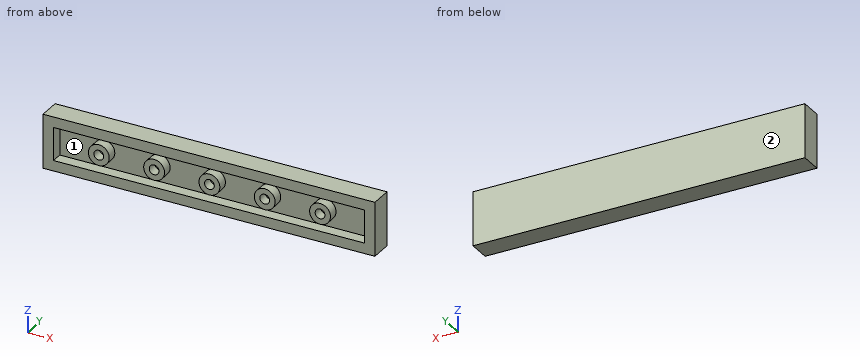
```python
from build123d import *

# Parameters (mm, degrees)
SKETCH1_W           = 47.75
SKETCH1_H           = 7.75
BOSS_EXTRUDE1_DEPTH = 3.15
SHELL1_T            = -1.5
SKETCH2_R           = 1.5
SKETCH2_R_2         = 0.7
BOSS_EXTRUDE2_DEPTH = 1.45


with BuildPart() as part:
    # Sketch1 → Boss-Extrude1 (new body)
    with BuildSketch(Plane(origin=(0, 0, 0), x_dir=(1, 0, 0), z_dir=(0, 1, 0))):
        Rectangle(SKETCH1_W, SKETCH1_H)
    extrude(amount=-BOSS_EXTRUDE1_DEPTH)

    # Shell1
    shell1_openings = [part.faces().sort_by_distance(p)[0] for p in [
        (0, -3.15, 0),
    ]]
    offset(amount=SHELL1_T, openings=shell1_openings, kind=Kind.INTERSECTION)

    # Sketch2 → Boss-Extrude2 (add)
    # profile 1 of 5: a face of its own
    with BuildSketch(Plane.XZ.offset(1.5)):
        with Locations(Location((-15.958333333, 0, 0), (0, 0, 90))):
            Circle(SKETCH2_R)
        with Locations(Location((-15.958333333, 0, 0), (0, 0, 90))):
            Circle(SKETCH2_R_2, mode=Mode.SUBTRACT)
    # profile 2 of 5: a face of its own
    with BuildSketch(Plane.XZ.offset(1.5)):
        with Locations(Location((-8, 0, 0), (0, 0, 90))):
            Circle(SKETCH2_R)
        with Locations(Location((-8, 0, 0), (0, 0, 90))):
            Circle(SKETCH2_R_2, mode=Mode.SUBTRACT)
    # profile 3 of 5: a face of its own
    with BuildSketch(Plane.XZ.offset(1.5)):
        with Locations(Location((-0.041666667, 0, 0), (0, 0, 90))):
            Circle(SKETCH2_R)
        with Locations(Location((-0.041666667, 0, 0), (0, 0, 90))):
            Circle(SKETCH2_R_2, mode=Mode.SUBTRACT)
    # profile 4 of 5: a face of its own
    with BuildSketch(Plane.XZ.offset(1.5)):
        with Locations(Location((7.916666667, 0, 0), (0, 0, 90))):
            Circle(SKETCH2_R)
        with Locations(Location((7.916666667, 0, 0), (0, 0, 90))):
            Circle(SKETCH2_R_2, mode=Mode.SUBTRACT)
    # profile 5 of 5: a face of its own
    with BuildSketch(Plane.XZ.offset(1.5)):
        with Locations(Location((15.875, 0, 0), (0, 0, 90))):
            Circle(SKETCH2_R)
        with Locations(Location((15.875, 0, 0), (0, 0, 90))):
            Circle(SKETCH2_R_2, mode=Mode.SUBTRACT)
    extrude(amount=BOSS_EXTRUDE2_DEPTH)


solid = part.part
```
For this review, take the finished solid that the model builds, in its own axes (mm). Face numbers are marked on the shaded views. Coordinates: 2 decimals unless noted, no trailing zeros. Loops run counter-clockwise (first coordinate to the right, second up) from the corner with the lowest first, then second, coordinate; pieces in that order, holes last. Notation, with made-up numbers: (48.25, 68.5) -> (105.25, 68.5) arc R21 cw to (105.25, 90.5) -> close; hole circle Ø3 at (68, 25.5). An arc over 180 degrees is marked (long way). Return JSON: item names as keys, results as strings. Group by question number.
(1) Mouldability with a two-part tool opening along X and no side actions: class the marked faces 1 and 2 as pulls with the +X half, pulls with the -X half, needs draft (parallel to the pull), parting line crosses it, or undercut.
(2) To check wall thickness, follow L1, parallel to Z at x = 0, y = -1.95 (3 decimals); L2, parallel to Z at x = -16.5, y = -2.3 (3 decimals); L3, parallel to X at y = -2.8, z = -2.25 (3 decimals). State the ranges of each line that lie inside material, in increasing order.
(3) Consider section B-B, the plane x = -8. Give the boundary of the cut face in (y, z) (3 decimals).
(4) Consider section A-A, the plane x = -13. Give the boundary of the cut face in (y, z) (3 decimals).
(5) For pin 1 Ø1.1 at (x, z) = (15.875, 0) entering from -Y; pin 2 Ø0.9 at (x, z) = (7.5, 0) entering from -Y, all flat-tipped, find the tip position at first contact; note any pin that passes through.
Results below:
{
 "1": {"face 1": "undercut", "face 2": "needs draft"},
 "2": {"L1": "z = -3.875 to -2.375, -1.499 to -0.699, 0.699 to 1.499, 2.375 to 3.875", "L2": "z = -3.875 to -2.375, -1.399 to -0.443, 0.443 to 1.399, 2.375 to 3.875", "L3": "x = -23.875 to -22.375, 22.375 to 23.875"},
 "3": {"outline": "(-3.15, -3.875) -> (0, -3.875) -> (0, 3.875) -> (-3.15, 3.875) -> (-3.15, 2.375) -> (-1.5, 2.375) -> (-1.5, 1.5) -> (-2.95, 1.5) -> (-2.95, 0.7) -> (-1.5, 0.7) -> (-1.5, -0.7) -> (-2.95, -0.7) -> (-2.95, -1.5) -> (-1.5, -1.5) -> (-1.5, -2.375) -> (-3.15, -2.375) -> close"},
 "4": {"outline": "(-3.15, -3.875) -> (0, -3.875) -> (0, 3.875) -> (-3.15, 3.875) -> (-3.15, 2.375) -> (-1.5, 2.375) -> (-1.5, -2.375) -> (-3.15, -2.375) -> close"},
 "5": {"pin 1": "stops at y = -1.5", "pin 2": "stops at y = -2.95"}
}
